Here's how the part is built. I have some questions about the finished solid (model axes, mm). A direction names the side the tool comes from. Round coordinates to 2 decimals unless told otherwise and drop trailing zeros. Loops run counter-clockwise (first coordinate to the right, second up) from the corner with the lowest first, then second, coordinate; pieces in that order, holes last. Notation, with made-up numbers: M -30,35.5 L 26,35.5 A16 ccw 26,65.5 Z; hole C -32,-17.75 d10. An arc over 180 degrees is marked long. Answer as a JSON object with one key per item and string values.
Autodesk Inventor part; units mm, degrees
ref_plane "YZ Plane" through (0, 0, 0) normal (1, 0, 0) x (0, 1, 0)
ref_plane "XZ Plane" through (0, 0, 0) normal (0, 1, 0) x (-1, 0, 0)
ref_plane "XY Plane" through (0, 0, 0) normal (0, 0, 1) x (1, 0, 0)
sketch "Sketch1" plane through (0, 0, 0) normal (0, 0, 1) x (1, 0, 0)
  circle A0 centre (0, 0) radius 33.655
  circle A1 centre (0, 0) radius 30.48
  dimension "d0" = 67.31
  dimension "d1" = 60.96
extrude "Extrusion1" add sketch "Sketch1" along normal blind 60.325
sketch "Sketch3" plane through (0, 0, 60.325) normal (0, 0, 1) x (1, 0, 0)
  line L0 (0, 0) -> (0, 30.48)
  circle A0 centre (0, 30.48) radius 1.27
  circle A1 centre (0, 30.48) radius 3.175
  circle A2 centre (-26.3965, 15.24) radius 3.175
  circle A3 centre (-26.3965, 15.24) radius 1.27
  circle A4 centre (-26.3965, -15.24) radius 3.175
  circle A5 centre (-26.3965, -15.24) radius 1.27
  circle A6 centre (0, -30.48) radius 3.175
  circle A7 centre (0, -30.48) radius 1.27
  circle A8 centre (26.3965, -15.24) radius 3.175
  circle A9 centre (26.3965, -15.24) radius 1.27
  circle A10 centre (26.3965, 15.24) radius 3.175
  circle A11 centre (26.3965, 15.24) radius 1.27
  dimension "d4" = 30.48
  dimension "d5" = 2.54
  dimension "d6" = 6.35
  dimension "d9" = 360
extrude "Extrusion2" add sketch "Sketch3" against normal up to surface (60.325 mm away)
extrude "Extrusion3" cut sketch "Sketch3" against normal up to surface (60.325 mm away) contours A0 | A3 | A5 | A7 | A9 | A11
properties part number "Spool" material "ABS Plastic"
Item 1: For P1, Ø12, axis at y = 11, z = 9, coming from the -X side; P2, Ø2, axis at x = 20, z = 43, coming from the -Y side; P3, Ø5, axis at y = -24, z = 11.5, coming from the -X side, each with a flat end and sliding along its axis, tell me the tip position at first contact or that it passes through.
Solution:
{"P1": "stops at x = -33.28", "P2": "stops at y = -27.78", "P3": "stops at x = -25.89"}
Item 2: I want a section at B-B on y = 22.5. List the corners of the cut face in (x, z) for me (3 decimals), plus the area to 3 significant figures.
Solution:
{"outline": "M -25.028,0 L -20.562,0 L -20.562,60.325 L -25.028,60.325 Z; M 20.562,0 L 25.028,0 L 25.028,60.325 L 20.562,60.325 Z", "area": "539 mm2"}
Item 3: I want a section at A-A on x = 0. List the corners of the cut face in (y, z) for me (3 decimals), plus the area to 3 significant figures.
Solution:
{"outline": "M -33.655,0 L -31.75,0 L -31.75,60.325 L -33.655,60.325 Z; M -29.21,0 L -27.305,0 L -27.305,60.325 L -29.21,60.325 Z; M 27.305,0 L 29.21,0 L 29.21,60.325 L 27.305,60.325 Z; M 31.75,0 L 33.655,0 L 33.655,60.325 L 31.75,60.325 Z", "area": "460 mm2"}
Item 4: If I drill on L1, parallel to X at y = -15, z = 31; L2, parallel to X at y = -15.24, z = 22.5; L3, parallel to Y at x = 1, z = 57.5, over which ranges is the centre line in solid material (lowest first)? Write a range as from..to.
Solution:
{"L1": "x = -30.13..-27.64, -25.15..-23.23, 23.23..25.15, 27.64..30.13", "L2": "x = -30.01..-27.67, -25.13..-23.22, 23.22..25.13, 27.67..30.01", "L3": "y = -33.64..-31.26, -29.7..-27.47, 27.47..29.7, 31.26..33.64"}
Item 5: I want a section at C-C on x = -15. List the corners of the cut face in (y, z) for me (3 decimals).
Solution:
{"outline": "M -30.127,0 L -26.534,0 L -26.534,60.325 L -30.127,60.325 Z; M 26.534,0 L 30.127,0 L 30.127,60.325 L 26.534,60.325 Z"}
Item 6: We'd pull the mould along Y, two halves only. Please class faces 1 (the face through (0.49, -33.65, 29.74)), 2 (the face through (-0.28, -31.72, 30.58)), 3 (the face through (-15.39, 26.31, 29.74)), 4 (the face through (25, 13, 0)): +Y half, -Y half, draft (parallel to the pull), parting line (faces both ways), or undercut.
Solution:
{"face 1": "-Y half", "face 2": "undercut", "face 3": "undercut", "face 4": "draft"}
Item 7: I want a section at D-D on z = 24. Count the separate pieces of the cut face and the enclosed holes in it, plus the area to 3 significant figures.
Solution:
{"separate pieces": "1", "enclosed holes": "7", "area": "702 mm2"}
Item 8: For faces 5 (the face through (-33.654, -0.246, 29.74)), 6 (the face through (15.39, -26.31, 29.74)), which set-ups out of +Z, -Z, +X, -X, +Y, -Y let a thin tool reach every point of the face, with its end or its side?
Solution:
{"face 5": "+Z, -Z, -X", "face 6": "+Z, -Z"}
